Autodesk Inventor part; units mm, degrees
ref_plane "MSC_PF1" through (0, 0, 0) normal (1, 0, 0) x (0, 1, 0)
ref_plane "MSC_PT1" through (0, 0, 0) normal (0, 0, -1) x (-1, 0, 0)
ref_plane "YZ Plane" through (0, 0, 0) normal (1, 0, 0) x (0, 1, 0)
sketch "Sketch1" plane through (0, 0, 0) normal (0, 1, 0) x (-1, 0, 0)
  point P0 (0, 0)
sketch "Sketch2" plane through (0, 0, 0) normal (0, 1, 0) x (-1, 0, 0)
  line L0 (-3, -25) -> (0, -25)
  line L1 (-3, -3.3) -> (-3, -25)
  line L2 (-6, -0.3) -> (-3, -3.3)
  line L3 (-6, 0) -> (-6, -0.3)
  line L4 (0, 0) -> (-6, 0)
  line L5 (0, -25) -> (0, 0)
  line L6 (0, -25) -> (0, 0)
  line L7 (0, -30) -> (0, 5)
  line L8 (1.2, 0) -> (-7.2, 0)
  dimension "d3" = 6
  dimension "d5" = 3
  dimension "d7" = 25
  dimension "ParC" = 0.3
  dimension "d22" = 0
  dimension "d23" = 0
  dimension "d43" = 45
revolve "Revolution1" add sketch "Sketch2" angle 360 about axis through (0, 0, -25) along (0, 0, -1)
sketch "Sketch3" plane through (0, 0, 0) normal (0, 0, 1) x (1, 0, 0)
  line L0 (-2, 1.1547) -> (-2, -1.1547)
  line L1 (0, 2.3094) -> (-2, 1.1547)
  line L2 (2, 1.1547) -> (0, 2.3094)
  line L3 (2, -1.1547) -> (2, 1.1547)
  line L4 (0, -2.3094) -> (2, -1.1547)
  line L5 (-2, -1.1547) -> (0, -2.3094)
  circle A0 centre (0, 0) radius 2 construction
  circle A1 centre (0, 0) radius 3 construction
  dimension "d11" = 4
  dimension "d13" = 120
  dimension "d15" = 120
extrude "Extrusion1" cut sketch "Sketch3" against normal blind 2.5
fillet "Fillet1" radius 0.3 1 edges at (-3, 0, -3.3)
chamfer "Chamfer1" distance 0.5 angle 45 1 edges at (-3, 0, -25) measured on face at (2.4612, -1.7154, -17.8081)
thread "Thread1"
ref_plane "MSC_PF1" through (0, 0, 0) normal (1, 0, 0) x (0, 1, 0)
ref_plane "MSC_PT1" through (0, 0, 0) normal (0, 0, -1) x (-1, 0, 0)
equation "\"d3\" = 0.5 * dk"
equation "\"d5\" = 0.5 * NND"
equation "\"d7\" = NLG"
equation "\"d43\" = 0.5 * ang"
equation "\"d18\" = r"
equation "\"d19\" = 0.5 * PTC"
equation "\"d39\" = 0.5 * PTC"
equation "\"d11\" = ParS"
equation "\"d16\" = ParT"
equation "\"NND\" = 6"
equation "\"PTC\" = 1"
equation "\"dk\" = 12"
equation "\"ParK\" = 3.3"
equation "\"ParS\" = 4"
equation "\"ParT\" = 2.5"
equation "\"r\" = 0.3"
equation "\"NLG\" = 25"
equation "\"ang\" = 90deg"
equation "\"THREADDIA\" = NND"
properties part number "CSK Allen Key 6x25mm" material "Steel, Mild"
CAD build for the part. Positions are in the model's coordinates, mm. A direction names the side the tool comes from. Coordinates: 2 decimals unless noted, no trailing zeros. Loops run counter-clockwise (first coordinate to the right, second up) from the corner with the lowest first, then second, coordinate; pieces in that order, holes last. Notation, with made-up numbers: (-4, 13.5) - (23, 13.5) arc R27 ccw to (23, 44.5) - close; hole circle Ø2 at (9.5, 36). An arc over 180 degrees is marked (long way). Use one line per item in the form item = value. Start each with the question number.
1) Tool access for faces 4 (the face through (-4.42, -4.06, -0.15)), 5 (the face through (2, 0, -1)): list every direction of +Z, -Z, +X, -X, +Y, -Y with a clear straight run to the whole face (end or side of a thin tool).
2) Flat gauge pins, fed straight in: pin 1 (6 mm diameter, centred on y = -1.5, z = -18.5, fed in from -X); pin 2 (6 mm diameter, centred on x = 1, z = -18, fed in from -Y); pin 3 (3 mm diameter, centred on x = 0, z = -13.5, fed in from +Y). Where does each tip first touch, or does it go through?
3) Drill centre lines: L1, parallel to Y at x = 0, z = -9.5; L2, parallel to Z at x = 2.75, y = -1.5; L3, parallel to Y at x = -1.75, z = -1.5. Where is each one in solid material? Low to high. Write a range as from..to.
4) Two-plate mould, pull along X, no slides. Class faces 1 (the face through (-2, 0, -1)), 2 (the face through (-3, 0, -14)), 3 (the face through (0, 0, -25)): +X half, -X half, draft (parallel to the pull), parting line (faces both ways), or undercut.
5) Band-saw the part on A-A (z = -18). Give the cut face in (x, y).
Check values:
q1.face_4 = +Z, -Z
q1.face_5 = +Z
q2.pin_1 = -3
q2.pin_2 = -3
q2.pin_3 = 3
q3.L1 = -3..3
q3.L2 = -3.17..0
q3.L3 = -4.47..-1.3, 1.3..4.47
q4.face_1 = undercut
q4.face_2 = parting line
q4.face_3 = draft
q5.outline = circle Ø6 at (0, 0)
